Build history of the part. All positions in model axes, mm. Give positions to 0.01 mm unless a question says otherwise; leave off trailing zeros. Order: outer loops, then holes, each group sorted by start corner. A loop starts at its lowest first (then second) coordinate and runs counter-clockwise, first axis right, second up. Notation, with made-up numbers: (62, 35.25) -> (114, 35.25) arc R14 ccw to (114, 60.25) -> close; hole circle Ø5 at (64.5, 28.5). An arc over 180 degrees is marked (long way). Write item = value, one per line. Start each with the question number.
Autodesk Inventor part; units mm, degrees
ref_plane "YZ Plane" through (0, 0, 0) normal (1, 0, 0) x (0, 1, 0)
ref_plane "XZ Plane" through (0, 0, 0) normal (0, 1, 0) x (-1, 0, 0)
ref_plane "XY Plane" through (0, 0, 0) normal (0, 0, 1) x (1, 0, 0)
sketch "スケッチ1" plane through (0, 0, 0) normal (0, 1, 0) x (-1, 0, 0)
  line L0 (-1.5, 0) -> (-1.5, 2.8)
  line L1 (-1.5, 2.8) -> (-2.25, 2.8)
  line L2 (-2.25, 2.8) -> (-2.25, 2.1)
  line L3 (-2.25, 2.1) -> (-3.1754, 2.1)
  line L4 (-3.1754, 2.1) -> (-3.1754, 0.2456)
  line L5 (-2.75, 0) -> (-1.5, 0)
  line L6 (-3.1754, 0.2456) -> (-2.75, 0)
  line L7 (0, -0.56) -> (0, 3.36)
  point P0 (0, 0)
  dimension "d0" = 2.75
  dimension "d1" = 3.1754
  dimension "d2" = 30
  dimension "d3" = 0.7
  dimension "d4" = 2.8
  dimension "d5" = 3
  dimension "d6" = 4.5
revolve "回転1" add sketch "スケッチ1" angle 360 about axis through (0, 0, -10) along (0, 0, 1)
sketch "スケッチ2" plane through (0, 0, 0) normal (0, 0, -1) x (-1, 0, 0)
  circle A0 centre (0, 0) radius 3.1754
  line L0 (0, 3.1754) -> (2.75, 1.5877)
  line L1 (2.75, 1.5877) -> (2.75, -1.5877)
  line L2 (2.75, -1.5877) -> (0, -3.1754)
  line L3 (0, -3.1754) -> (-2.75, -1.5877)
  line L4 (-2.75, -1.5877) -> (-2.75, 1.5877)
  line L5 (-2.75, 1.5877) -> (0, 3.1754)
  point P0 (0, -3.1754)
  point P1 (0, -3.1754)
extrude "押し出し1" cut sketch "スケッチ2" against normal through all contours A0 L1 | L0 A0 | A0 L2 | L5 A0 | A0 L3 | L4 A0
chamfer "面取り1" distance 0.3 angle 45 6 edges at (0, 3.1754, 1.1728) (-2.75, 1.5877, 1.1728) (2.75, 1.5877, 1.1728) (2.75, -1.5877, 1.1728) (0, -3.1754, 1.1728) (-2.75, -1.5877, 1.1728)
thread "ねじ1"
properties part number "S3-07-3W" material "チタン"
(1) Wall check: line 1 (Y direction, x = 0, z = 2.2); line 2 (Y direction, x = 0, z = 1.1); line 3 (Z direction, x = 0.75, y = 2.25). Give the ranges that are in metal, low to high. Write a range as [from, to].
(2) Cut at C-C, the plane z = 2.3. Give the cut face in (x, y).
(3) Flat gauge pins, fed straight in: P1, Ø1.5, axis at x = 1.5, z = 1, coming from the +Y side; P2, Ø2, axis at x = 1.5, y = 0.5, coming from the -Z side. Where does each tip first touch, or does it go through?
(4) Cut at A-A, the plane x = 0. Give the cut face in (y, z), plus the area to 3 significant figures.
(5) Mould opens along X. For faces 1 (the face through (-0.29, -2.23, 2.45)), 2 (the face through (-1.5, 0.07, 1.42)), 3 (the face through (-2.52, -1.42, 0.08)), 4 (the face through (1.391, 2.373, 1.035)) say: released by +X, released by -X, zero draft, split by the parting line, or undercut.
(6) Cut at B-B, the plane z = 1.3. Give the cut face in (x, y).
Results:
q1.line_1 = [-2.25, -1.5], [1.5, 2.25]
q1.line_2 = [-3.03, -1.5], [1.5, 3.03]
q1.line_3 = [0, 2.1]
q2.outline = circle Ø4.5 at (0, 0); hole circle Ø3 at (0, 0)
q3.P1 = 2.74
q3.P2 = 0
q4.outline = (-3.03, 0.16) -> (-2.75, 0) -> (-1.5, 0) -> (-1.5, 2.8) -> (-2.25, 2.8) -> (-2.25, 2.1) -> (-3.03, 2.1) -> close; (1.5, 0) -> (2.75, 0) -> (3.03, 0.16) -> (3.03, 2.1) -> (2.25, 2.1) -> (2.25, 2.8) -> (1.5, 2.8) -> close
q4.area = 7.41 mm2
q5.face_1 = split by the parting line
q5.face_2 = undercut
q5.face_3 = released by -X
q5.face_4 = released by +X
q6.outline = (-2.75, -1.29) -> (-2.49, -1.74) -> (-0.26, -3.03) -> (0.26, -3.03) -> (2.49, -1.74) -> (2.75, -1.29) -> (2.75, 1.29) -> (2.49, 1.74) -> (0.26, 3.03) -> (-0.26, 3.03) -> (-2.49, 1.74) -> (-2.75, 1.29) -> close; hole circle Ø3 at (0, 0)
